from build123d import *

# Parameters (mm, degrees)
BOSS_EXTRUDE1_DEPTH    = 1.8
LATCH_DEPTH            = 2
LPATTERN1_COUNT        = 2
LPATTERN1_PITCH        = 15.5
LPATTERN1_COPY_1_DEPTH = 2
LPATTERN2_COUNT        = 2
LPATTERN2_PITCH        = 15.5
LPATTERN2_COPY_1_DEPTH = 2


with BuildPart() as part:
    # Sketch1 → Boss-Extrude1 (new body)
    with BuildSketch(Plane.XY):
        with BuildLine():
            Line((-21.23, 10.12), (-21.23, -10.12))
            ThreePointArc((-21.23, -10.12), (-20.679360749, -11.449360749), (-19.35, -12))
            Line((-19.35, -12), (19.35, -12))
            ThreePointArc((19.35, -12), (20.679360749, -11.449360749), (21.23, -10.12))
            Line((21.23, -10.12), (21.23, 10.12))
            ThreePointArc((21.23, 10.12), (20.679360749, 11.449360749), (19.35, 12))
            Line((19.35, 12), (-19.35, 12))
            ThreePointArc((-19.35, 12), (-20.679360749, 11.449360749), (-21.23, 10.12))
        make_face()
    extrude(amount=BOSS_EXTRUDE1_DEPTH)

    # Sketch4 → Latch (add, symmetric)
    with BuildSketch(Plane(origin=(0, 0, 0), x_dir=(0, 0, -1), z_dir=(1, 0, 0))):
        Polygon((-1.4, 12), (-0.938119785, 12.8), (-0.4, 12.8), (-0.4, 12), align=None)
    latch = extrude(amount=LATCH_DEPTH, both=True)

    # Mirror1: Latch across plane
    add(latch.mirror(Plane.ZX))

    # LPattern1: Latch ×2
    with Locations(*[(i * LPATTERN1_PITCH, 0, 0) for i in range(1, LPATTERN1_COUNT)]):
        add(latch)

    # LPattern1 copy 1 sketch → LPattern1 copy 1 (add, symmetric)
    with BuildSketch(Plane(origin=(15.5, 0, 0), x_dir=(0, 0, -1), z_dir=(1, 0, 0))):
        Polygon((-1.4, -12), (-0.938119785, -12.8), (-0.4, -12.8), (-0.4, -12), align=None)
    extrude(amount=LPATTERN1_COPY_1_DEPTH, both=True)

    # LPattern2: Latch ×2
    with Locations(*[(-i * LPATTERN2_PITCH, 0, 0) for i in range(1, LPATTERN2_COUNT)]):
        add(latch)

    # LPattern2 copy 1 sketch → LPattern2 copy 1 (add, symmetric)
    with BuildSketch(Plane(origin=(-15.5, 0, 0), x_dir=(0, 0, -1), z_dir=(1, 0, 0))):
        Polygon((-1.4, -12), (-0.938119785, -12.8), (-0.4, -12.8), (-0.4, -12), align=None)
    extrude(amount=LPATTERN2_COPY_1_DEPTH, both=True)


solid = part.part
Here's how the part is built. I have some questions about the finished solid (model axes, mm). A direction names the side the tool comes from. Coordinates: 2 decimals unless noted, no trailing zeros. Order: outer loops, then holes, each group sorted by start corner. A loop starts at its lowest first (then second) coordinate and runs counter-clockwise, first axis right, second up. Notation, with made-up numbers: M 8,83.5 L 33,83.5 A17 cw 33,96.5 Z; hole C -20,22 d6. An arc over 180 degrees is marked long. Answer as CSV lines item,"result". Start each with the question number.
1. I need wall thicknesses on line 1 (Y direction, x = 11, z = 0.65); line 2 (X direction, y = 11.75, z = 0.35); line 3 (X direction, y = 11, z = 1.1). Which ranges of each line are inside material? Lowest first, please. Write a range as [from, to].
2. I want a section at B-B, the plane x = 12.5. Write out the boundary of the cut face in (y, z).
3. For pin 1 (0.9 mm diameter, centred on y = -12.5, z = 1, fed in from +X); pin 2 (0.9 mm diameter, centred on x = 1, y = 12.5, fed in from -Z); pin 3 (0.9 mm diameter, centred on y = 12.5, z = 1, fed in from -X), each with a flat end and sliding along its axis, tell me the tip position at first contact or that it passes through.
4. We'd pull the mould along X, two halves only. Please class faces 1 (the flat face through (0.028, 12.394, 1.172)), 2 (the flat face through (-13.5, 12.4, 0.8)), 3 (the flat face through (-17.5, -12.4, 0.8)): released by +X, released by -X, zero draft, split by the parting line, or undercut.
5. On a 3-axis mill with a long thin cutter (end or side, diameter ignored), from which of +Z, -Z, +X, -X, +Y, -Y can I reach the whole of each face in a straight line? I mean faces 4 (the flat face through (-13.5, -12.4, 0.8)), 5 (the flat face through (2, 12.4, 0.8)), 6 (the flat face through (0, -12.4, 0.4)), 7 (the flat face through (0, 12.4, 0.4)), 8 (the flat face through (-17.5, 12.4, 0.8)). Say none if no direction works.
6. I want a section at A-A, the plane x = 1. Write out the boundary of the cut face in (y, z), and give its area (3 significant figures).
Recorded:
1,line 1,"y = [-12, 12]"
1,line 2,"x = [-20.29, 20.29]"
1,line 3,"x = [-21.01, 21.01]"
2,outline,"M -12,0 L 12,0 L 12,1.8 L -12,1.8 Z"
3,pin 1,"stops at x = 17.5"
3,pin 2,"stops at z = 0.4"
3,pin 3,"stops at x = -17.5"
4,face 1,"zero draft"
4,face 2,"undercut"
4,face 3,"released by -X"
5,face 4,"+Z, -Z, -Y"
5,face 5,"+Z, -Z, +Y"
5,face 6,"-Z, +X, -X, -Y"
5,face 7,"-Z, +X, -X, +Y"
5,face 8,"+Z, -Z, -X, +Y"
6,outline,"M -12.8,0.4 L -12,0.4 L -12,0 L 12,0 L 12,0.4 L 12.8,0.4 L 12.8,0.94 L 12,1.4 L 12,1.8 L -12,1.8 L -12,1.4 L -12.8,0.94 Z"
6,area,"44.4 mm2"
